Verification items for the finished model (mm, model axes). A direction names the side the tool comes from. Coordinates: 2 decimals unless noted, no trailing zeros. Order: outer loops, then holes, each group sorted by start corner. A loop starts at its lowest first (then second) coordinate and runs counter-clockwise, first axis right, second up. Notation, with made-up numbers: (6.25, 21.5) - (64.25, 21.5) arc R28 cw to (64.25, 49.5) - close; hole circle Ø10 at (53.5, 77). An arc over 180 degrees is marked (long way). Answer as CSV lines item,"result". Start each with the question number.
1. Section check C-C (y = 0.75). Record the cut outline in (x, z), and give its area (3 significant figures).
2. Set-up check for faces 5 (the flat face through (10, 3.175, 53)), 6 (the flat face through (20, 3, 3)), 7 (the flat face through (12, 3, 28)): record each of +Z, -Z, +X, -X, +Y, -Y from which the full face is reachable in a straight line by a thin tool's end or side.
3. Section check A-A (x = 13). Record the cut outline in (y, z) (3 decimals), and give its area (3 significant figures).
4. Go/stop test with flat-tipped pins: pin 1 (3 mm diameter, centred on y = 1.5, z = 21.5, fed in from +X); pin 2 (1.5 mm diameter, centred on x = 3.5, y = 4, fed in from +Z); pin 3 (7.5 mm diameter, centred on x = 13.5, z = 54, fed in from +Y) (3 decimals). Record where each tip stops, or that it passes through.
5. Mould release check, pull along Z, two halves, no side actions. Record for faces 1 (the flat face through (4, 3, 17)), 2 (the flat face through (20, 2, 41)), 3 (the flat face through (10, 5, 45)), 4 (the flat face through (12, 3, 5)): pulls with the +Z half, pulls with the -Z half, needs draft (parallel to the pull), parting line crosses it, or undercut.
6. Section check D-D (x = 10). Record the cut outline in (y, z) (3 decimals), and give its area (3 significant figures).
7. Section check B-B (z = 30.5). Record the cut outline in (x, y).
8. Material ranges on L1, parallel to Z at x = 10, y = 1.75; L2, parallel to Z at x = 14.25, y = 5.75; L3, parallel to Z at x = 15.75, y = 2.25, recorded low to high. Write a range as [from, to].
from build123d import *

# Parameters (mm, degrees)
SKETCH2_W             = 20
SKETCH2_H             = 60
BOSS_EXTRUDE1_DEPTH   = 6.35
SKETCH4_W             = 16
SKETCH4_H             = 23
CUT_EXTRUDE1_DEPTH    = 64.563531211
M2_CLEARANCE_HOLE1_D  = 2.4
SKETCH10_W            = 15
SKETCH10_H            = 3.175
CUT_EXTRUDE2_DEPTH    = 64.563531211
F_2_CLEARANCE_HOLE1_D = 2.4384


with BuildPart() as part:
    # Sketch2 → Boss-Extrude1 (new body)
    with BuildSketch(Plane(origin=(0, 0, 0), x_dir=(1, 0, 0), z_dir=(0, 1, 0))):
        with Locations((10, -30)):
            Rectangle(SKETCH2_W, SKETCH2_H)
    extrude(amount=BOSS_EXTRUDE1_DEPTH)

    # Sketch4 → Cut-Extrude1 (cut, through all)
    with BuildSketch(Plane(origin=(0, 6.35, 0), x_dir=(1, 0, 0), z_dir=(0, 1, 0))):
        with Locations((12, -16.5)):
            Rectangle(SKETCH4_W, SKETCH4_H)
    extrude(amount=-CUT_EXTRUDE1_DEPTH, mode=Mode.SUBTRACT)

    # M2 Clearance Hole1 (through all)
    with Locations(Plane(origin=(0, 6.35, 0), x_dir=(1, 0, 0), z_dir=(0, 1, 0))):
        with Locations((10, -30.5), (10, -2.5)):
            Hole(M2_CLEARANCE_HOLE1_D / 2)

    # Sketch10 → Cut-Extrude2 (cut, through all)
    with BuildSketch(Plane(origin=(20, 0, 0), x_dir=(0, 0, -1), z_dir=(1, 0, 0))):
        with Locations((-52.5, 4.7625)):
            Rectangle(SKETCH10_W, SKETCH10_H)
    extrude(amount=-CUT_EXTRUDE2_DEPTH, mode=Mode.SUBTRACT)

    # #2 Clearance Hole1 (through all)
    with Locations(Plane(origin=(0, 3.175, 0), x_dir=(1, 0, 0), z_dir=(0, 1, 0))):
        with Locations((4.803847577, -48), (15.196152423, -48), (10, -57)):
            Hole(F_2_CLEARANCE_HOLE1_D / 2)


solid = part.part
Evaluation:
1,outline,"(0, 0) - (20, 0) - (20, 5) - (4, 5) - (4, 28) - (20, 28) - (20, 60) - (0, 60) - close; hole circle Ø2.44 at (4.8, 48); hole circle Ø2.44 at (10, 57); hole circle Ø2.4 at (10, 2.5); hole circle Ø2.4 at (10, 30.5); hole circle Ø2.44 at (15.2, 48)"
1,area,"809 mm²"
2,face 5,"+Z, +X, -X, +Y"
2,face 6,"+Z, -Z, +X, +Y, -Y"
2,face 7,"+X, +Y, -Y"
3,outline,"(0, 0) - (6.35, 0) - (6.35, 5) - (0, 5) - close; (0, 28) - (6.35, 28) - (6.35, 45) - (3.175, 45) - (3.175, 60) - (0, 60) - close"
3,area,"187 mm²"
4,pin 1,"stops at x = 4"
4,pin 2,"stops at z = 45"
4,pin 3,"stops at y = 3.175"
5,face 1,"undercut"
5,face 2,"needs draft"
5,face 3,"pulls with the +Z half"
5,face 4,"undercut"
6,outline,"(0, 0) - (6.35, 0) - (6.35, 1.3) - (0, 1.3) - close; (0, 3.7) - (6.35, 3.7) - (6.35, 5) - (0, 5) - close; (0, 28) - (6.35, 28) - (6.35, 29.3) - (0, 29.3) - close; (0, 31.7) - (6.35, 31.7) - (6.35, 45) - (3.175, 45) - (3.175, 55.781) - (0, 55.781) - close; (0, 58.219) - (3.175, 58.219) - (3.175, 60) - (0, 60) - close"
6,area,"149 mm²"
7,outline,"(0, 0) - (8.8, 0) - (8.8, 6.35) - (0, 6.35) - close; (11.2, 0) - (20, 0) - (20, 6.35) - (11.2, 6.35) - close"
8,L1,"z = [0, 1.3], [3.7, 5], [28, 29.3], [31.7, 55.78], [58.22, 60]"
8,L2,"z = [0, 5], [28, 45]"
8,L3,"z = [0, 5], [28, 46.91], [49.09, 60]"
